Geometry: final body of the model. Coordinates: model frame, mm. A direction names the side the tool comes from. Coordinates: 2 decimals unless noted, no trailing zeros. Order: outer loops, then holes, each group sorted by start corner. A loop starts at its lowest first (then second) coordinate and runs counter-clockwise, first axis right, second up. Notation, with made-up numbers: (-25, 32) - (10, 32) arc R34 ccw to (10, 62) - close; hole circle Ø7 at (-25.75, 34). An arc over 180 degrees is marked (long way). Use a Markdown table: item, result. Add a question column.
```python
from build123d import *

# Parameters (mm, degrees)
SKETCH_1_R        = 7
SKETCH_1_R_2      = 5.65
EXTRUDE_1_DEPTH   = 4
SKETCH_1_R_3      = 5.75
EXTRUDE_1_2_DEPTH = 4
SKETCH_1_R_4      = 6
EXTRUDE_1_3_DEPTH = 4
EXTRUDE_2_DEPTH   = 1


with BuildPart() as part:
    # Sketch 1 → Extrude 1 (new body)
    with BuildSketch(Plane(origin=(0, 0, 0), x_dir=(1, 0, 0), z_dir=(0, 1, 0))):
        with Locations((-73.735173333, 44.289748166)):
            Circle(SKETCH_1_R)
        with Locations((-73.735173333, 44.289748166)):
            Circle(SKETCH_1_R_2, mode=Mode.SUBTRACT)
    extrude(amount=EXTRUDE_1_DEPTH)



with BuildPart() as body_2:
    # Sketch 1 → Extrude 1 2 (new body)
    with BuildSketch(Plane(origin=(0, 0, 0), x_dir=(1, 0, 0), z_dir=(0, 1, 0))):
        with Locations((-49.788051119, 44.289748166)):
            Circle(SKETCH_1_R)
        with Locations((-49.788051119, 44.289748166)):
            Circle(SKETCH_1_R_3, mode=Mode.SUBTRACT)
    extrude(amount=EXTRUDE_1_2_DEPTH)


with BuildPart() as body_3:
    # Sketch 1 → Extrude 1 3 (new body)
    with BuildSketch(Plane(origin=(0, 0, 0), x_dir=(1, 0, 0), z_dir=(0, 1, 0))):
        with Locations((-62.341002405, 63.939282004)):
            Circle(SKETCH_1_R)
        with Locations((-62.341002405, 63.939282004)):
            Circle(SKETCH_1_R_4, mode=Mode.SUBTRACT)
    extrude(amount=EXTRUDE_1_3_DEPTH)


with BuildPart() as part_1:
    add(part.part)

    add(body_2.part)  # Extrude 2 merges body 2

    add(body_3.part)  # Extrude 2 merges body 3
    # Sketch 2 → Extrude 2 (add)
    with BuildSketch(Plane(origin=(0, 0, 0), x_dir=(1, 0, 0), z_dir=(0, 1, 0))):
        Polygon((-66.735173333, 44.289748166), (-56.743768428, 45.075875842), (-56.371981746, 43.565889762), (-67.1134612, 42.842031358), align=None)
        Polygon((-59.44276594, 57.567451388), (-55.341606688, 48.550971059), (-53.588038725, 49.751237508), (-57.6700519, 58.725624806), align=None)
    extrude(amount=EXTRUDE_2_DEPTH)


solid = part_1.part
```
1) Section query A-A (z = -39.5). Return the cut outline in (x, y).
2) Section query B-B (x = -47). Return the cut outline in (y, z).
3) Access query for faces 4 (the flat face through (-62, 1, -44)), 5 (the flat face through (-61.809, 0.493, -44.677)), 6 (the cylindrical face through (-43.32, 1.97, -41.61)). Directions: +Z, -Z, +X, -X, +Y, -Y. A direction counts if a zero-diameter tool reaches every point of the face in a straight line with its end or side. Return the directions, or none.
4) Section query C-C (y = 1.9). Return the cut outline in (x, z).
5) Section query D-D (x = -63). Return the cut outline in (y, z).
6) Line query: line 1 (X direction, y = 0.3, z = -44); line 2 (X direction, y = 1.75, z = -45.5); line 3 (X direction, y = 3.5, z = -43.5). Output: solid intervals per line, ascending. Write a range as from..to.
7) First-contact query: pin 1 (1 mm diameter, centred on x = -47.5, y = 2, fed in from -Z); pin 2 (12 mm diameter, centred on x = -74, z = -42.5, fed in from -Y); pin 3 (1.8 mm diameter, centred on x = -60.5, z = -43.5, fed in from +Y); pin 4 (1 mm diameter, centred on y = 2, z = -49.5, fed in from -X). Flat tips, straight axial feed; report the tip coordinate or a pass-through.
8) Draft query along Z for faces 1 (the flat face through (-57, 1, -54)), 2 (the flat face through (-61.745, 0.493, -43.204)), 3 (the flat face through (-57, 0, -54)). Return one class per face: released by +Z, released by -Z, zero draft, split by the parting line, or undercut.
From the geometry:
| question | item | result |
|---|---|---|
| 1 | outline | (-78.84, 0) - (-76.73, 0) - (-76.73, 4) - (-78.84, 4) - close; (-70.74, 0) - (-68.63, 0) - (-68.63, 4) - (-70.74, 4) - close; (-54.89, 0) - (-52.97, 0) - (-52.97, 4) - (-54.89, 4) - close; (-46.61, 0) - (-44.68, 0) - (-44.68, 4) - (-46.61, 4) - close |
| 2 | outline | (0, -50.71) - (4, -50.71) - (4, -49.32) - (0, -49.32) - close; (0, -39.26) - (4, -39.26) - (4, -37.87) - (0, -37.87) - close |
| 3 | face 4 | +Z, +Y |
| 3 | face 5 | +Y, -Y |
| 3 | face 6 | +Y |
| 4 | outline | circle Ø14 at (-73.74, -44.29); circle Ø14 at (-62.34, -63.94); circle Ø14 at (-49.79, -44.29); hole circle Ø11.3 at (-73.74, -44.29); hole circle Ø12 at (-62.34, -63.94); hole circle Ø11.5 at (-49.79, -44.29) |
| 5 | outline | (0, -70.91) - (4, -70.91) - (4, -69.9) - (0, -69.9) - close; (0, -57.98) - (4, -57.98) - (4, -56.97) - (0, -56.97) - close; (0, -44.58) - (1, -44.58) - (1, -43.12) - (0, -43.12) - close |
| 6 | line 1 | x = -80.73..-79.38, -68.09..-55.53, -44.05..-42.79 |
| 6 | line 2 | x = -80.63..-79.25, -68.22..-66.84, -56.68..-55.41, -44.17..-42.89 |
| 6 | line 3 | x = -80.69..-79.33, -68.14..-66.78, -56.74..-55.48, -44.09..-42.83 |
| 7 | pin 1 | stops at z = -51.06 |
| 7 | pin 2 | stops at y = 0 |
| 7 | pin 3 | stops at y = 1 |
| 7 | pin 4 | stops at x = -78.91 |
| 8 | face 1 | undercut |
| 8 | face 2 | released by +Z |
| 8 | face 3 | zero draft |
